For this review, use the dimensioned drawing (mm, ordinates from the lowest corner) and the shaded views. Give positions to 0.01 mm unless a question says otherwise; leave off trailing zeros. Loops run counter-clockwise (first coordinate to the right, second up) from the corner with the lowest first, then second, coordinate; pieces in that order, holes last. Notation, with made-up numbers: (26, 84) - (38, 84) arc R29 ccw to (38, 106) - close; hole circle Ø5 at (-21, -6). An arc over 180 degrees is marked (long way). Put each result on its own line as item: value.
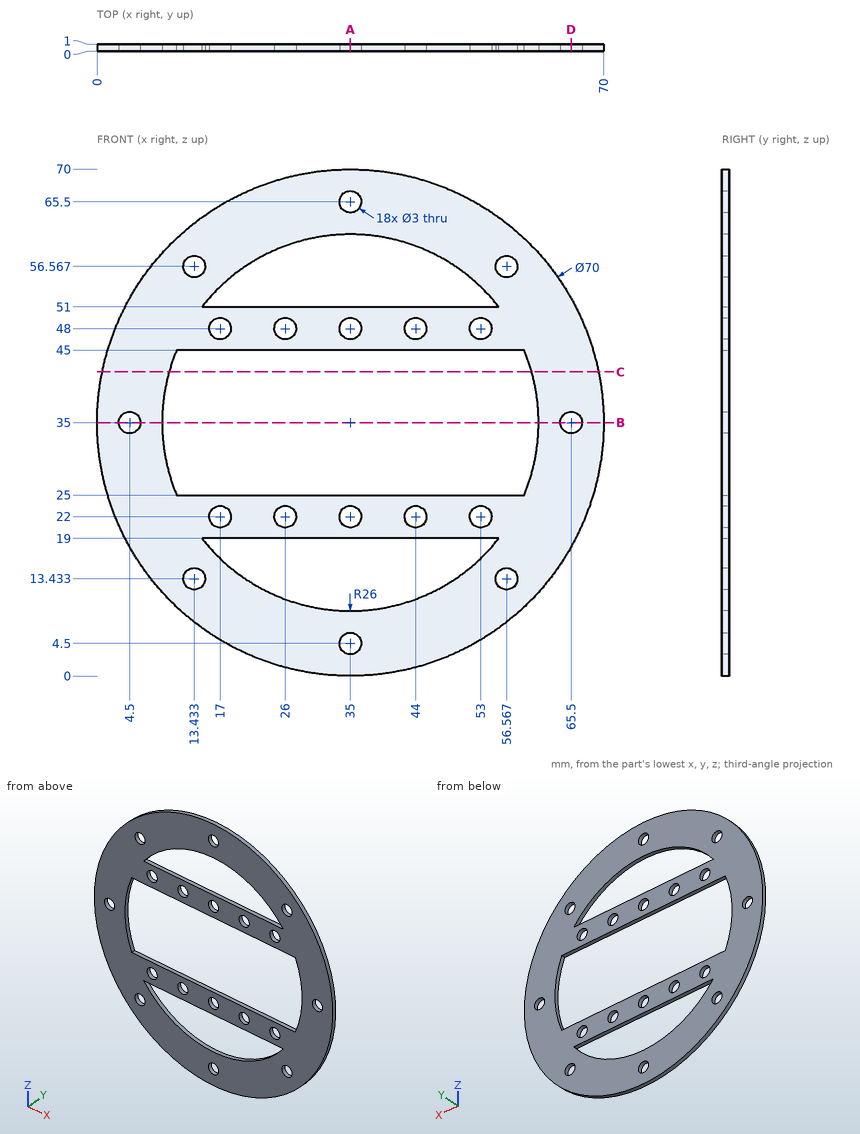
1) Take a section at C-C on z = 42. State the section outline as (x, y) points, and give its area (3 significant figures).
Geometry check:
outline: (0.71, 0) - (9.96, 0) - (9.96, 1) - (0.71, 1) - close; (60.04, 0) - (69.29, 0) - (69.29, 1) - (60.04, 1) - close
area: 18.5 mm²
2) Take a section at D-D on x = 65.5. State the section outline as (y, z) points.
Geometry check:
outline: (0, 17.83) - (1, 17.83) - (1, 33.5) - (0, 33.5) - close; (0, 36.5) - (1, 36.5) - (1, 52.17) - (0, 52.17) - close
3) Insertion check: pin 1 Ø0.5 at (x, y) = (44, 0.5) entering from +Z. The pin has a flat end and moves straight along its axis. Give the tip position at first contact, or say it passes through.
Geometry check:
pin 1: stops at z = 68.89
4) Take a section at A-A on x = 35. State how many separate pieces and enclosed holes the cut face has, and give its area (3 significant figures).
Geometry check:
separate pieces: 8
enclosed holes: 0
area: 18.0 mm²
5) Take a section at B-B on z = 35. State the section outline as (x, y) points.
Geometry check:
outline: (0, 0) - (3, 0) - (3, 1) - (0, 1) - close; (6, 0) - (9, 0) - (9, 1) - (6, 1) - close; (61, 0) - (64, 0) - (64, 1) - (61, 1) - close; (67, 0) - (70, 0) - (70, 1) - (67, 1) - close
6) Wall thickness on line 1 (Z direction, x = 29, y = 0.85); line 2 (X direction, y = 0.6, z = 22); line 3 (X direction, y = 0.25, z = 35): over which ranges is each line inside the solid? List them lowest first.
Geometry check:
line 1: z = 0.52 to 9.7, 19 to 25, 45 to 51, 60.3 to 69.48
line 2: x = 2.5 to 15.5, 18.5 to 24.5, 27.5 to 33.5, 36.5 to 42.5, 45.5 to 51.5, 54.5 to 67.5
line 3: x = 0 to 3, 6 to 9, 61 to 64, 67 to 70
